Build history of the part. All positions in model axes, mm. Face numbers are marked on the shaded views. A direction names the side the tool comes from. Give positions to 0.01 mm unless a question says otherwise; leave off trailing zeros. Order: outer loops, then holes, each group sorted by start corner. A loop starts at its lowest first (then second) coordinate and runs counter-clockwise, first axis right, second up. Notation, with made-up numbers: (36, -36.75) -> (42, -36.75) arc R13 ccw to (42, -32.75) -> close; hole circle Ø11 at (-37.75, -35). An arc over 180 degrees is marked (long way). One line per item, written item: value. Start each with the question number.
(1) Saw through at B-B on z = 5.5. Give the cut face in (x, y).
(2) Saw through at C-C on x = 23. Give the cut face in (y, z), plus the area to 3 significant figures.
(3) Two-plate mould, pull along X, no slides. Class the marked faces 4, 5 and 6: +X half, -X half, draft (parallel to the pull), parting line (faces both ways), or undercut.
(4) Saw through at A-A on z = 28.5. Count the separate pieces of the cut face and the enclosed holes in it, plus the area to 3 significant figures.
(5) Pin check, flat tips, straight feed: pin 1 (12 mm diameter, centred on x = -30.5, z = 27, fed in from -Y); pin 2 (1.5 mm diameter, centred on y = -6.5, z = 23, fed in from +X); pin 3 (1.6 mm diameter, centred on y = -29, z = 14.5, fed in from +X). Stop position of each tip, or through.
(6) Which spindle directions (+Z, -Z, +X, -X, +Y, -Y) get a long thin tool onto all of the face, cutting with end or side? Do the marked faces 1, 2 and 3. Say none if no direction does.
(7) Saw through at D-D on y = 6. Give the cut face in (x, z).
(8) Probe line 1 (Y direction, x = -42.5, z = 13); line 2 (X direction, y = 32, z = 26); line 3 (Z direction, x = 14, y = 4.5). List the from-to ranges inside material, lowest first.
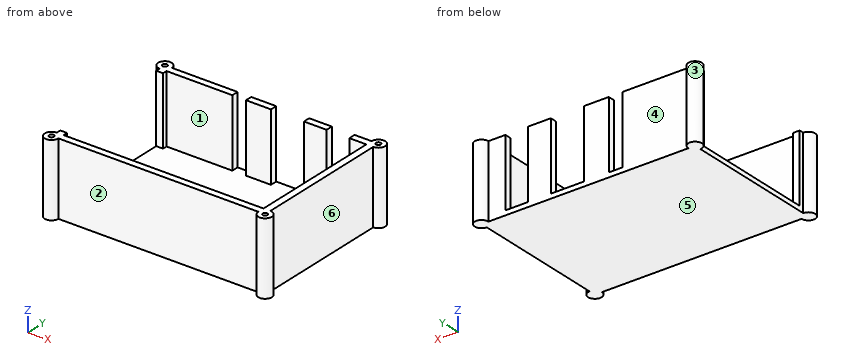
```python
from build123d import *

# Parameters (mm, degrees)
F1_DEPTH = 32
F3_DEPTH = 30
F5_D     = 2.1
F5_DEPTH = 10
F5_TIP   = 0.63090365


with BuildPart() as f1:
    # F0 (on Top) → F1 (new body)
    with BuildSketch(Plane.XY):
        with BuildLine():
            Line((-44, -32.5), (44, -32.5))
            ThreePointArc((44, -32.5), (49.1213203436, -34.6213203436), (47, -29.5))
            Line((47, -29.5), (47, 29.5))
            ThreePointArc((47, 29.5), (49.1213203436, 34.6213203436), (44, 32.5))
            Line((44, 32.5), (-44, 32.5))
            ThreePointArc((-44, 32.5), (-49.1213203436, 34.6213203436), (-47, 29.5))
            Line((-47, 29.5), (-47, -29.5))
            ThreePointArc((-47, -29.5), (-49.1213203436, -34.6213203436), (-44, -32.5))
        make_face()
    extrude(amount=F1_DEPTH)

    # F2 (on face) → F3 (cut)
    with BuildSketch(Plane.XY.offset(32)):
        Polygon((44, -29.5), (44, 29.5), (36.5, 29.5), (36.5, 32.5), (26.5, 32.5), (26.5, 29.5), (16.5, 29.5), (16.5, 32.5), (2, 32.5), (2, 29.5), (-9, 29.5), (-9, 32.5), (-15, 32.5), (-15, 29.5), (-44, 29.5), (-44, 27.5), (-47, 27.5), (-47, -27.5), (-44, -27.5), (-44, -29.5), align=None)
    extrude(amount=-F3_DEPTH, mode=Mode.SUBTRACT)

    # F5
    with Locations(Plane.XY.offset(32)):
        with Locations((-47, 32.5), (47, 32.5), (47, -32.5), (-47, -32.5)):
            Hole(F5_D / 2, depth=F5_DEPTH)
            with Locations((0, 0, -(F5_DEPTH + F5_TIP / 2))):  # 118° drill point
                Cone(0, F5_D / 2, F5_TIP, mode=Mode.SUBTRACT)


solid = f1.part
```
Results below:
1. outline: (-47, -29.5) arc R3 ccw (long way) to (-44, -32.5) -> (44, -32.5) arc R3 ccw (long way) to (47, -29.5) -> (47, 29.5) arc R3 ccw (long way) to (44, 32.5) -> (36.5, 32.5) -> (36.5, 29.5) -> (44, 29.5) -> (44, -29.5) -> (-44, -29.5) -> (-44, -27.5) -> (-47, -27.5) -> close; (-47, 27.5) -> (-44, 27.5) -> (-44, 29.5) -> (-15, 29.5) -> (-15, 32.5) -> (-44, 32.5) arc R3 ccw (long way) to (-47, 29.5) -> close; (-9, 29.5) -> (2, 29.5) -> (2, 32.5) -> (-9, 32.5) -> close; (16.5, 29.5) -> (26.5, 29.5) -> (26.5, 32.5) -> (16.5, 32.5) -> close
2. outline: (-32.5, 0) -> (32.5, 0) -> (32.5, 32) -> (29.5, 32) -> (29.5, 2) -> (-29.5, 2) -> (-29.5, 32) -> (-32.5, 32) -> close
2. area: 310 mm²
3. face 4: undercut
3. face 5: draft
3. face 6: +X half
4. separate pieces: 4
4. enclosed holes: 4
4. area: 732 mm²
5. pin 1: stops at y = -32.5
5. pin 2: stops at x = 47
5. pin 3: stops at x = 48.31
6. face 1: +Z
6. face 2: +Z, -Z, -Y
6. face 3: +Z, -Z
7. outline: (-47, 0) -> (47, 0) -> (47, 32) -> (44, 32) -> (44, 2) -> (-47, 2) -> close
8. line 1: y = -32.5 to -29.5, 29.5 to 32.5
8. line 2: x = -49.96 to -47.92, -46.08 to -15, -9 to 2, 16.5 to 26.5, 36.5 to 46.08, 47.92 to 49.96
8. line 3: z = 0 to 2
